Source: CAD feature listing. Evaluate the final solid. Frame: model axes, mm. Round coordinates to 2 decimals unless told otherwise and drop trailing zeros. Answer as CSV lines item,"result".
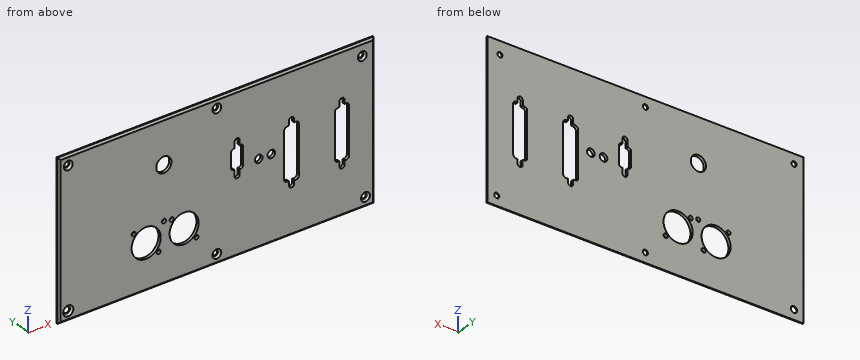
from build123d import *

# Parameters (mm, degrees)
F0_W     = 250
F0_H     = 120
F0_R     = 2.5
F0_R_2   = 1.6
F0_R_3   = 11.5
F0_R_4   = 2
F0_R_5   = 6
F0_R_6   = 3
F1_DEPTH = 2.29
F2_SIZE  = 1.5
F3_SIZE  = 1.5


with BuildPart() as f1:
    # F0 (on Front) → F1 (new body)
    with BuildSketch(Plane.XZ):
        with Locations((7.931469, 14.123547)):
            Rectangle(F0_W, F0_H)
        with Locations((-109.568531, -38.376453)):
            Circle(F0_R, mode=Mode.SUBTRACT)
        with Locations((-38.056882, -20.8)):
            Circle(F0_R_2, mode=Mode.SUBTRACT)
        with Locations((-8.056882, -20.8)):
            Circle(F0_R_2, mode=Mode.SUBTRACT)
        with Locations((-57.856882, -1)):
            Circle(F0_R_2, mode=Mode.SUBTRACT)
        with Locations((-47.956882, -10.9)):
            Circle(F0_R_3, mode=Mode.SUBTRACT)
        with Locations((-27.856882, -1)):
            Circle(F0_R_2, mode=Mode.SUBTRACT)
        with Locations((-17.956882, -10.9)):
            Circle(F0_R_3, mode=Mode.SUBTRACT)
        with Locations((-33.856882, 0)):
            Circle(F0_R_2, mode=Mode.SUBTRACT)
        with Locations((7.931469, -38.376453)):
            Circle(F0_R_4, mode=Mode.SUBTRACT)
        with Locations((125.431469, -38.376453)):
            Circle(F0_R_4, mode=Mode.SUBTRACT)
        with Locations((-33.969466, 40.677104)):
            Circle(F0_R_5, mode=Mode.SUBTRACT)
        with Locations((-109.568531, 66.623547)):
            Circle(F0_R_4, mode=Mode.SUBTRACT)
        with Locations((7.931, 66.623547)):
            Circle(F0_R_4, mode=Mode.SUBTRACT)
        with BuildLine():
            ThreePointArc((26.514029, 33.811025), (27.948503, 33.513178), (28.784517, 32.310053))
            Line((28.784517, 32.310053), (28.784517, 17.936876))
            ThreePointArc((28.784517, 17.936876), (27.93903, 16.743219), (26.503268, 16.463479))
            Line((26.503268, 16.463479), (26.034518, 16.552957))
            Line((26.034518, 16.552957), (26.034518, 12.623465))
            ThreePointArc((26.034518, 12.623465), (24.034518, 10.623465), (22.034518, 12.623465))
            Line((22.034518, 12.623465), (22.034518, 17.316499))
            Line((22.034518, 17.316499), (20.786522, 17.554723))
            ThreePointArc((20.786522, 17.554723), (19.704803, 18.196975), (19.284518, 19.38271))
            Line((19.284518, 19.38271), (19.284518, 31.38271))
            ThreePointArc((19.284518, 31.38271), (20.085689, 32.371468), (21.251265, 32.882302))
            Line((21.251265, 32.882302), (22.034518, 33.020524))
            Line((22.034518, 33.020524), (22.034518, 37.623465))
            ThreePointArc((22.034518, 37.623465), (24.034518, 39.623465), (26.034518, 37.623465))
            Line((26.034518, 37.623465), (26.034518, 33.726406))
            Line((26.034518, 33.726406), (26.514029, 33.811025))
        make_face(mode=Mode.SUBTRACT)
        with Locations((41.034031, 18.623465)):
            Circle(F0_R_6, mode=Mode.SUBTRACT)
        with Locations((51.034031, 18.623465)):
            Circle(F0_R_6, mode=Mode.SUBTRACT)
        with BuildLine():
            ThreePointArc((69.034518, -9.181223), (67.034518, -11.181223), (65.034518, -9.181223))
            Line((65.034518, -9.181223), (65.034518, -5.865349))
            Line((65.034518, -5.865349), (62.965224, -5.522281))
            ThreePointArc((62.965224, -5.522281), (61.605659, -5.014743), (61.034518, -3.680648))
            Line((61.034518, -3.680648), (61.034031, -2.680648))
            Line((61.034031, -2.680648), (61.034031, 31.319352))
            ThreePointArc((61.034031, 31.319352), (61.537051, 32.945268), (62.870351, 34.00307))
            Line((62.870351, 34.00307), (65.034705, 34.40553))
            Line((65.034705, 34.40553), (65.034705, 37.791433))
            ThreePointArc((65.034705, 37.791433), (67.007175, 39.81859), (69.034331, 37.846121))
            Line((69.034331, 37.846121), (69.071112, 35.156098))
            Line((69.071112, 35.156098), (69.850695, 35.301061))
            ThreePointArc((69.850695, 35.301061), (72.196438, 34.615273), (73.034031, 32.319352))
            Line((73.034031, 32.319352), (73.034031, -3.680648))
            ThreePointArc((73.034031, -3.680648), (72.193258, -5.958464), (69.870961, -6.667181))
            Line((69.870961, -6.667181), (69.034518, -6.528508))
            Line((69.034518, -6.528508), (69.034518, -9.181223))
        make_face(mode=Mode.SUBTRACT)
        with BuildLine():
            ThreePointArc((108.977516, -9.376453), (106.977516, -11.376453), (104.977516, -9.376453))
            Line((104.977516, -9.376453), (104.977516, -6.064618))
            Line((104.977516, -6.064618), (104.977516, -5.563356))
            Line((104.977516, -5.563356), (102.935548, -5.224819))
            ThreePointArc((102.935548, -5.224819), (101.80013, -4.549377), (101.423057, -3.283197))
            Line((101.423057, -3.283197), (101.412046, 30.7371))
            Line((101.412046, 30.7371), (101.411781, 31.557157))
            ThreePointArc((101.411781, 31.557157), (101.773775, 32.651359), (102.717343, 33.313175))
            Line((102.717343, 33.313175), (104.889253, 33.717688))
            Line((104.889253, 33.717688), (104.889253, 34.211154))
            Line((104.889253, 34.211154), (104.889253, 37.623547))
            ThreePointArc((104.889253, 37.623547), (106.889253, 39.623547), (108.889253, 37.623547))
            Line((108.889253, 37.623547), (108.889253, 34.960369))
            Line((108.889253, 34.960369), (108.889253, 34.441248))
            Line((108.889253, 34.441248), (109.822674, 34.615095))
            ThreePointArc((109.822674, 34.615095), (111.757696, 34.035583), (112.411415, 32.124355))
            Line((112.411415, 32.124355), (112.423064, -3.875644))
            ThreePointArc((112.423064, -3.875644), (111.661619, -5.670743), (109.841285, -6.369719))
            Line((109.841285, -6.369719), (108.977516, -6.226515))
            Line((108.977516, -6.226515), (108.977516, -6.727777))
            Line((108.977516, -6.727777), (108.977516, -9.376453))
        make_face(mode=Mode.SUBTRACT)
        with Locations((122.931469, 64.123547)):
            Circle(F0_R_4, mode=Mode.SUBTRACT)
    extrude(amount=F1_DEPTH)

    # F2
    f2_edges = [f1.edges().sort_by_distance(p)[0] for p in [
        (-117.068531, -2.29, 14.123547),
        (7.931469, -2.29, -45.876453),
        (132.931469, -2.29, 14.123547),
        (7.931469, -2.29, 74.123547),
    ]]
    chamfer(f2_edges, length=F2_SIZE)

    # F3
    f3_edges = [f1.edges().sort_by_distance(p)[0] for p in [
        (-111.568531, -2.29, 66.623547),
        (5.931, -2.29, 66.623547),
        (120.931469, -2.29, 64.123547),
        (123.431469, -2.29, -38.376453),
        (5.931469, -2.29, -38.376453),
        (-112.068531, -2.29, -38.376453),
    ]]
    chamfer(f3_edges, length=F3_SIZE)


solid = f1.part
1. Section query A-A on y = -1.75. Give the number of separate pieces and of enclosed holes in the cut face, and give its area (3 significant figures).
Results below:
separate pieces,"1"
enclosed holes,"19"
area,"26,900 mm2"
2. Line query: L1, parallel to X at y = -1.1, z = -15.5; L2, parallel to Z at x = -58, y = -1.4; L3, parallel to X at y = -1.4, z = -18. Output: solid intervals per line, ascending. Write a range as [from, to].
Results below:
L1,"[-116.76, -58.5], [-37.42, -28.5], [-7.42, 132.62]"
L2,"[-45.27, -16.5], [-5.3, -2.59], [0.59, 73.51]"
L3,"[-116.46, -57], [-38.91, -27], [-8.91, 132.32]"
3. Pin query (flat end, axial travel): pin 1 (0.7 mm diameter, centred on y = -1.5, z = 12.5, fed in from -X); pin 2 (1.1 mm diameter, centred on y = -1.5, z = 35.5, fed in from -X); pin 3 (0.7 mm diameter, centred on y = -1.5, z = 31, fed in from +X). Return the tip coordinate at first contact, or that it passes through.
Results below:
pin 1,"x = -116.71"
pin 2,"x = -116.91"
pin 3,"x = 132.57"
